Input: part model. Units: mm. Frame: model coordinates. A direction names the side the tool comes from. Round coordinates to 2 decimals unless told otherwise and drop trailing zeros. Order: outer loops, then holes, each group sorted by start corner. A loop starts at its lowest first (then second) coordinate and runs counter-clockwise, first axis right, second up. Notation, with made-up numbers: (81, 77.5) -> (109, 77.5) arc R31 ccw to (109, 107.5) -> close; hole circle Ø3 at (-29.5, -18). An arc over 180 degrees is marked (long way). Use a Markdown table: item, result.
Autodesk Inventor part; units mm, degrees
ref_plane "YZ Plane" through (0, 0, 0) normal (1, 0, 0) x (0, 1, 0)
ref_plane "XZ Plane" through (0, 0, 0) normal (0, 1, 0) x (-1, 0, 0)
ref_plane "XY Plane" through (0, 0, 0) normal (0, 0, 1) x (1, 0, 0)
sketch "Sketch1" plane through (0, 0, 0) normal (0, 0, 1) x (1, 0, 0)
  line L0 (-4.8, 0) -> (0.8, 0) construction
  line L1 (0, -56) -> (0, 56) construction
  line L2 (-4, 40) -> (0, 40)
  line L3 (0, 40) -> (0, -40)
  line L4 (0, -40) -> (-4, -40)
  line L5 (-4, -40) -> (-4, 40)
  line L6 (-1.5443, -40) -> (-4, -20)
  point P0 (0, 0)
  dimension "d0" = 8
  dimension "d1" = 80
  dimension "d13" = 20
  dimension "d14" = 3.0886
  dimension "d17" = 7
revolve "Revolution1" add sketch "Sketch1" angle 360 about axis through (0, 40, 0) along (0, -1, 0) contours L2 L3 L4 L6 L5
sketch "Sketch2" plane through (0, 40, 0) normal (0, 1, 0) x (1, 0, 0)
  circle A0 centre (0, 0) radius 4
hole "Hole1" at (0, 40, 0) direction (0, -1, 0) diameter 3.242 depth 15 tip angle 118
chamfer "Chamfer1" distance 0.25 angle 45 2 edges at (1.5443, -40, 0) (4, 40, 0)
properties part number "FCT-01-001C" material "Aço SAE 1045"
1) Ray query, probe 1 along Z at (x, y) = (0, 31); probe 2 along Z at (x, y) = (-1.25, 36.5). Return the intervals inside material, ascending.
Answer key:
| item | result |
|---|---|
| probe 1 | z = -4 to -1.62, 1.62 to 4 |
| probe 2 | z = -3.8 to -1.03, 1.03 to 3.8 |
2) Set-up query: faces 4 (the face through (0, -40, 0)), 5 (the face through (1.438, 32.395, 0.748)). Return all of +Z, -Z, +X, -X, +Y, -Y with unobstructed straight access to the full face (end or side cutting, diameter ignored); none if empty.
Answer key:
| item | result |
|---|---|
| face 4 | +Z, -Z, +X, -X, -Y |
| face 5 | +Y |
3) Contact query for flat-ended pins moving along their axis: P1, Ø2.5, axis at x = 0, z = 0, coming from the +Y side; P2, Ø4, axis at x = 3, y = -16.5, coming from the +Z side; P3, Ø3, axis at x = 0, z = -1.5, coming from the -Y side; P4, Ø3, axis at x = 0.5, z = 3, coming from the -Y side. Output: stop coordinate, or through.
Answer key:
| item | result |
|---|---|
| P1 | stops at y = 24.78 |
| P2 | stops at z = 3.87 |
| P3 | stops at y = -40 |
| P4 | stops at y = -39.78 |
4) Cut plane A-A on y = 30.5. Return loops of the section in (x, z), and give its area (3 significant figures).
Answer key:
| item | result |
|---|---|
| outline | circle Ø8 at (0, 0); hole circle Ø3.24 at (0, 0) |
| area | 42.0 mm^2 |
5) Draft query along Z for faces 1 (the face through (-1, 40, 2)), 2 (the face through (-0.275, 24.195, -0.061)), 3 (the face through (0.867, 10.293, -3.905)). Return one class per face: released by +Z, released by -Z, zero draft, split by the parting line, or undercut.
Answer key:
| item | result |
|---|---|
| face 1 | zero draft |
| face 2 | undercut |
| face 3 | split by the parting line |
6) Cut plane B-B on y = 11.5. Return loops of the section in (x, z).
Answer key:
| item | result |
|---|---|
| outline | circle Ø8 at (0, 0) |
